Geometry: final body of the model. Coordinates: model frame, mm. Face numbers are marked on the shaded views. Round coordinates to 2 decimals unless told otherwise and drop trailing zeros. Order: outer loops, then holes, each group sorted by start corner. A loop starts at its lowest first (then second) coordinate and runs counter-clockwise, first axis right, second up. Notation, with made-up numbers: (89.25, -23.5) - (135.25, -23.5) arc R7 cw to (135.25, -17.5) - close; hole circle Ø10 at (72.25, 14). An arc over 180 degrees is marked (long way). Put each result on its own line as item: value. Start each with the question number.
(1) Material intervals for L1, parallel to Y at x = 6, z = 1; L2, parallel to X at y = -1, z = -0.5; L3, parallel to X at y = -2.25, z = 0, sorted ascending. Write a range as [from, to].
(2) Section A-A (z = 0). Output: boundary loops of the cut face in (x, y), and give its area (3 significant figures).
(3) Pull-direction query (Z, two-part tool) for the marked faces 1, 2, 3 and 4; classes: released by +Z, released by -Z, zero draft, split by the parting line, or undercut.
(4) Section C-C (x = 23). Output: boundary loops of the cut face in (y, z).
(5) Pin query (flat end, axial travel): P1, Ø1, axis at x = 8.5, z = -3, coming from the -Y side; P2, Ø4, axis at x = 12, y = -2, coming from the +Z side; P3, Ø1, axis at x = 20, z = 2, coming from the -Y side. Return the tip coordinate at first contact, or that it passes through.
(6) Section B-B (x = 6). Output: boundary loops of the cut face in (y, z), and give its area (3 significant figures).
(7) Section D-D (x = 52.88). Output: boundary loops of the cut face in (y, z).
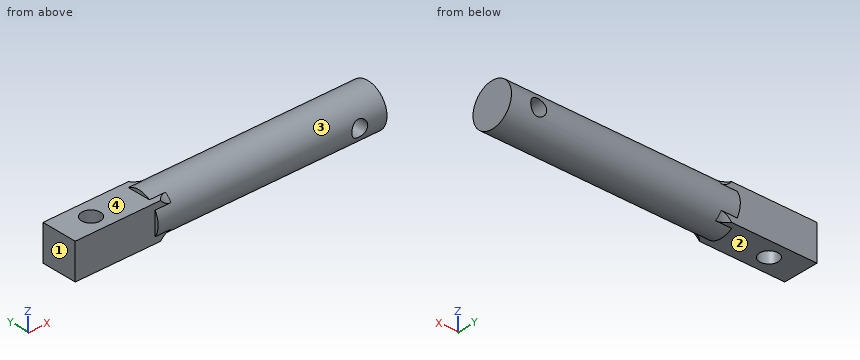
from build123d import *

# Parameters (mm, degrees)
ESQUISSE1_W                  = 6.7
ESQUISSE1_H                  = 6.7
BOSS_EXTRU_1_DEPTH           = 15
ESQUISSE2_R                  = 4
BOSS_EXTRU_2_DEPTH           = 43
ENL_V_MAT_EXTRU_1_DEPTH      = 59.275209137
ENL_V_MAT_EXTRU_1_DEPTH_BACK = 59.275209137
ESQUISSE3_R                  = 1.5
CONG_1_R                     = 3
ENL_V_MAT_EXTRU_2_DEPTH      = 59.600533392
ENL_V_MAT_EXTRU_2_DEPTH_BACK = 59.600533392
ESQUISSE4_R                  = 1.75


with BuildPart() as part:
    # Esquisse1 → Boss.-Extru.1 (new body)
    with BuildSketch(Plane.YZ):
        Rectangle(ESQUISSE1_W, ESQUISSE1_H)
    extrude(amount=BOSS_EXTRU_1_DEPTH)

    # Esquisse2 → Boss.-Extru.2 (add)
    with BuildSketch(Plane.YZ.offset(15)):
        with Locations(Location((0, 0, 0), (0, 0, 56.877059792))):
            Circle(ESQUISSE2_R)
    extrude(amount=BOSS_EXTRU_2_DEPTH)

    # Esquisse3 → Enlèv. mat.-Extru.1 (cut, two sides: drawn at the far end of the back side and taken through both)
    with BuildSketch(Plane(origin=(0, 0, 0), x_dir=(-1, 0, 0), z_dir=(0, 1, 0)).offset(-ENL_V_MAT_EXTRU_1_DEPTH_BACK)):
        with Locations(Location((-52.88, 0, 0), (0, 0, 90))):
            Circle(ESQUISSE3_R)
    extrude(amount=ENL_V_MAT_EXTRU_1_DEPTH + ENL_V_MAT_EXTRU_1_DEPTH_BACK, mode=Mode.SUBTRACT)

    # Congé1
    # the kernel refuses this fillet: 3 mm, written as the material it adds along each edge
    with BuildSketch(Plane(origin=(15, 0, 0), x_dir=(0, -0.9627373172303846, -0.27043827024302985), z_dir=(0, -0.27043827024302985, 0.9627373172303846))) as cong_1_piece_1_section:
        with BuildLine():
            CenterArc((4 + CONG_1_R, CONG_1_R), CONG_1_R, 180, 90)
            Line((4 + CONG_1_R, 0), (4, 0))
            Line((4, 0), (4, CONG_1_R))
        make_face()
    cong_1_piece_1 = revolve(axis=Axis((15, 0, 0), (1, 0, 0)), revolution_arc=238.619303718, mode=Mode.PRIVATE)
    cong_1_piece_1 = split(cong_1_piece_1, bisect_by=Plane(origin=(16.010494669, -2.96099487, 3.35), z_dir=(0, 0, -1)), keep=Keep.TOP, mode=Mode.PRIVATE)
    cong_1_piece_1 = split(cong_1_piece_1, bisect_by=Plane(origin=(16.010494669, -2.96099487, -3.35), z_dir=(0, 0, 1)), keep=Keep.TOP, mode=Mode.PRIVATE)
    cong_1_piece_1 = split(cong_1_piece_1, bisect_by=Plane(origin=(16.010494669, 3.35, -2.96099477), z_dir=(0, -1, 0)), keep=Keep.TOP, mode=Mode.PRIVATE)
    cong_1_piece_1 = split(cong_1_piece_1, bisect_by=Plane(origin=(16.010494669, -3.35, -2.96099477), z_dir=(0, 1, 0)), keep=Keep.TOP, mode=Mode.PRIVATE)
    add(cong_1_piece_1)
    with BuildSketch(Plane(origin=(15, 0, 0), x_dir=(0, 0.27043827024295675, -0.962737317230405), z_dir=(0, -0.962737317230405, -0.27043827024295675))) as cong_1_piece_2_section:
        with BuildLine():
            CenterArc((4 + CONG_1_R, CONG_1_R), CONG_1_R, 180, 90)
            Line((4 + CONG_1_R, 0), (4, 0))
            Line((4, 0), (4, CONG_1_R))
        make_face()
    cong_1_piece_2 = revolve(axis=Axis((15, 0, 0), (1, 0, 0)), revolution_arc=238.619303718, mode=Mode.PRIVATE)
    cong_1_piece_2 = split(cong_1_piece_2, bisect_by=Plane(origin=(16.010494669, 2.96099477, 3.35), z_dir=(0, 0, -1)), keep=Keep.TOP, mode=Mode.PRIVATE)
    cong_1_piece_2 = split(cong_1_piece_2, bisect_by=Plane(origin=(16.010494669, 2.96099477, -3.35), z_dir=(0, 0, 1)), keep=Keep.TOP, mode=Mode.PRIVATE)
    cong_1_piece_2 = split(cong_1_piece_2, bisect_by=Plane(origin=(16.010494669, 3.35, -2.96099487), z_dir=(0, -1, 0)), keep=Keep.TOP, mode=Mode.PRIVATE)
    cong_1_piece_2 = split(cong_1_piece_2, bisect_by=Plane(origin=(16.010494669, -3.35, -2.96099487), z_dir=(0, 1, 0)), keep=Keep.TOP, mode=Mode.PRIVATE)
    add(cong_1_piece_2)
    with BuildSketch(Plane(origin=(15, 0, 0), x_dir=(0, 0.9627373172304061, 0.27043827024295286), z_dir=(0, 0.27043827024295286, -0.9627373172304061))) as cong_1_piece_3_section:
        with BuildLine():
            CenterArc((4 + CONG_1_R, CONG_1_R), CONG_1_R, 180, 90)
            Line((4 + CONG_1_R, 0), (4, 0))
            Line((4, 0), (4, CONG_1_R))
        make_face()
    cong_1_piece_3 = revolve(axis=Axis((15, 0, 0), (1, 0, 0)), revolution_arc=238.619303718, mode=Mode.PRIVATE)
    cong_1_piece_3 = split(cong_1_piece_3, bisect_by=Plane(origin=(16.010494669, 2.96099487, 3.35), z_dir=(0, 0, -1)), keep=Keep.TOP, mode=Mode.PRIVATE)
    cong_1_piece_3 = split(cong_1_piece_3, bisect_by=Plane(origin=(16.010494669, 2.96099487, -3.35), z_dir=(0, 0, 1)), keep=Keep.TOP, mode=Mode.PRIVATE)
    cong_1_piece_3 = split(cong_1_piece_3, bisect_by=Plane(origin=(16.010494669, 3.35, 2.96099477), z_dir=(0, -1, 0)), keep=Keep.TOP, mode=Mode.PRIVATE)
    cong_1_piece_3 = split(cong_1_piece_3, bisect_by=Plane(origin=(16.010494669, -3.35, 2.96099477), z_dir=(0, 1, 0)), keep=Keep.TOP, mode=Mode.PRIVATE)
    add(cong_1_piece_3)
    with BuildSketch(Plane(origin=(15, 0, 0), x_dir=(0, -0.2704382702430083, 0.9627373172303906), z_dir=(0, 0.9627373172303906, 0.2704382702430083))) as cong_1_piece_4_section:
        with BuildLine():
            CenterArc((4 + CONG_1_R, CONG_1_R), CONG_1_R, 180, 90)
            Line((4 + CONG_1_R, 0), (4, 0))
            Line((4, 0), (4, CONG_1_R))
        make_face()
    cong_1_piece_4 = revolve(axis=Axis((15, 0, 0), (1, 0, 0)), revolution_arc=238.619303718, mode=Mode.PRIVATE)
    cong_1_piece_4 = split(cong_1_piece_4, bisect_by=Plane(origin=(16.010494669, -2.96099477, 3.35), z_dir=(0, 0, -1)), keep=Keep.TOP, mode=Mode.PRIVATE)
    cong_1_piece_4 = split(cong_1_piece_4, bisect_by=Plane(origin=(16.010494669, -2.96099477, -3.35), z_dir=(0, 0, 1)), keep=Keep.TOP, mode=Mode.PRIVATE)
    cong_1_piece_4 = split(cong_1_piece_4, bisect_by=Plane(origin=(16.010494669, 3.35, 2.96099487), z_dir=(0, -1, 0)), keep=Keep.TOP, mode=Mode.PRIVATE)
    cong_1_piece_4 = split(cong_1_piece_4, bisect_by=Plane(origin=(16.010494669, -3.35, 2.96099487), z_dir=(0, 1, 0)), keep=Keep.TOP, mode=Mode.PRIVATE)
    add(cong_1_piece_4)

    # Esquisse4 → Enlèv. mat.-Extru.2 (cut, two sides: drawn at the far end of the back side and taken through both)
    with BuildSketch(Plane(origin=(0, 0, 3.35), x_dir=(-1, 0, 0), z_dir=(0, 0, -1)).offset(-ENL_V_MAT_EXTRU_2_DEPTH_BACK)):
        with Locations(Location((-6, 0, 0), (0, 0, 180))):
            Circle(ESQUISSE4_R)
    extrude(amount=ENL_V_MAT_EXTRU_2_DEPTH + ENL_V_MAT_EXTRU_2_DEPTH_BACK, mode=Mode.SUBTRACT)


solid = part.part
Checks:
1. L1: y = [-3.35, -1.75], [1.75, 3.35]
1. L2: x = [0, 4.56], [7.44, 51.47], [54.29, 58]
1. L3: x = [0, 51.38], [54.38, 58]
2. outline: (0, -3.35) - (15, -3.35) - (15, -4) - (51.38, -4) - (51.38, 4) - (15, 4) - (15, 3.35) - (0, 3.35) - close; (54.38, -4) - (58, -4) - (58, 4) - (54.38, 4) - close; hole circle Ø3.5 at (6, 0)
2. area: 411 mm²
3. face 1: zero draft
3. face 2: released by -Z
3. face 3: split by the parting line
3. face 4: released by +Z
4. outline: circle Ø8 at (0, 0)
5. P1: stops at y = -3.35
5. P2: stops at z = 3.35
5. P3: stops at y = -3.71
6. outline: (-3.35, -3.35) - (-1.75, -3.35) - (-1.75, 3.35) - (-3.35, 3.35) - close; (1.75, -3.35) - (3.35, -3.35) - (3.35, 3.35) - (1.75, 3.35) - close
6. area: 21.4 mm²
7. outline: (-3.71, -1.5) arc R4 ccw to (3.71, -1.5) - close; (-3.71, 1.5) - (3.71, 1.5) arc R4 ccw to start
